Here's how the part is built. I have some questions about the finished solid (model axes, mm). Face numbers are marked on the shaded views. A direction names the side the tool comes from. Give positions to 0.01 mm unless a question says otherwise; leave off trailing zeros. Loops run counter-clockwise (first coordinate to the right, second up) from the corner with the lowest first, then second, coordinate; pieces in that order, holes last. Notation, with made-up numbers: (68.25, 23) - (88.25, 23) arc R25 ccw to (88.25, 36) - close; hole circle Ø6 at (26.5, 48). An arc over 180 degrees is marked (long way). Use a Markdown table: item, result.
from build123d import *

# Parameters (mm, degrees)
F1_R     = 28.05
F1_R_2   = 6.55
F2_DEPTH = 5
F3_SIZE  = 1
F5_DEPTH = 5.001


with BuildPart() as f2:
    # F1 (on Top) → F2 (new body)
    with BuildSketch(Plane.XY):
        Circle(F1_R)
        Circle(F1_R_2, mode=Mode.SUBTRACT)
    extrude(amount=F2_DEPTH)

    # F3
    f3_edges = [f2.edges().sort_by_distance(p)[0] for p in [
        (-28.05, 0, 0),
        (-28.05, 0, 5),
        (-6.55, 0, 5),
        (-6.55, 0, 0),
    ]]
    chamfer(f3_edges, length=F3_SIZE)

    # F4 (on face) → F5 (cut, through all)
    with BuildSketch(Plane.XY.offset(5)):
        with BuildLine():
            Line((4.0373102115, 9.746929068), (9.2035365484, 22.2193027569))
            ThreePointArc((9.2035365484, 22.2193027569), (0, 24.05), (-9.2035365484, 22.2193027569))
            Line((-9.2035365484, 22.2193027569), (-4.0373102115, 9.746929068))
            ThreePointArc((-4.0373102115, 9.746929068), (0, 10.55), (4.0373102115, 9.746929068))
        make_face()
        with BuildLine():
            ThreePointArc((-14.6407123677, 19.080147834), (-20.827910961, 12.025), (-23.844248916, 3.1391549229))
            Line((-23.844248916, 3.1391549229), (-10.4597432875, 1.3770513279))
            ThreePointArc((-10.4597432875, 1.3770513279), (-9.1365680099, 5.275), (-6.422433076, 8.3698777401))
            Line((-6.422433076, 8.3698777401), (-14.6407123677, 19.080147834))
        make_face()
        with BuildLine():
            ThreePointArc((-23.844248916, -3.1391549229), (-20.827910961, -12.025), (-14.6407123677, -19.080147834))
            Line((-14.6407123677, -19.080147834), (-6.422433076, -8.3698777401))
            ThreePointArc((-6.422433076, -8.3698777401), (-9.1365680099, -5.275), (-10.4597432875, -1.3770513279))
            Line((-10.4597432875, -1.3770513279), (-23.844248916, -3.1391549229))
        make_face()
        with BuildLine():
            ThreePointArc((-9.2035365484, -22.2193027569), (0, -24.05), (9.2035365484, -22.2193027569))
            Line((9.2035365484, -22.2193027569), (4.0373102115, -9.746929068))
            ThreePointArc((4.0373102115, -9.746929068), (0, -10.55), (-4.0373102115, -9.746929068))
            Line((-4.0373102115, -9.746929068), (-9.2035365484, -22.2193027569))
        make_face()
        with BuildLine():
            ThreePointArc((14.6407123677, -19.080147834), (20.827910961, -12.025), (23.844248916, -3.1391549229))
            Line((23.844248916, -3.1391549229), (10.4597432875, -1.3770513279))
            ThreePointArc((10.4597432875, -1.3770513279), (9.1365680099, -5.275), (6.422433076, -8.3698777401))
            Line((6.422433076, -8.3698777401), (14.6407123677, -19.080147834))
        make_face()
        with BuildLine():
            ThreePointArc((23.844248916, 3.1391549229), (20.827910961, 12.025), (14.6407123677, 19.080147834))
            Line((14.6407123677, 19.080147834), (6.422433076, 8.3698777401))
            ThreePointArc((6.422433076, 8.3698777401), (9.1365680099, 5.275), (10.4597432875, 1.3770513279))
            Line((10.4597432875, 1.3770513279), (23.844248916, 3.1391549229))
        make_face()
    extrude(amount=-F5_DEPTH, mode=Mode.SUBTRACT)


solid = f2.part
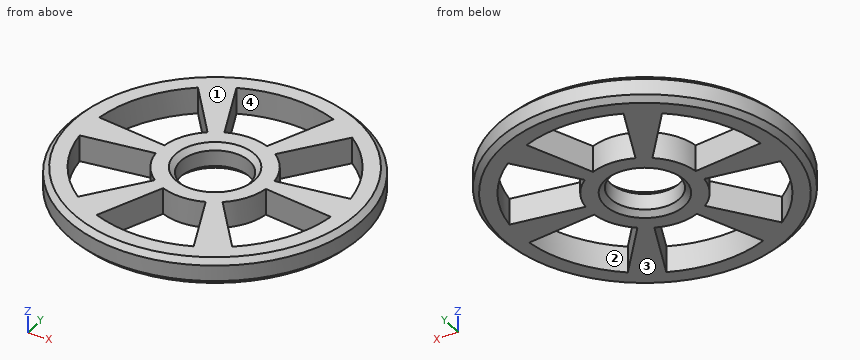
(1) Suppose I cut it at C-C on y = 0. Write out the boundary of the cut face in (x, z).
A:
| item | result |
|---|---|
| outline | (-28.05, 1) - (-27.05, 0) - (-7.55, 0) - (-6.55, 1) - (-6.55, 4) - (-7.55, 5) - (-27.05, 5) - (-28.05, 4) - close; (6.55, 1) - (7.55, 0) - (27.05, 0) - (28.05, 1) - (28.05, 4) - (27.05, 5) - (7.55, 5) - (6.55, 4) - close |
(2) If I drill on line 1 (Y direction, x = 0, z = 2.35); line 2 (Y direction, x = 15, z = 2.5); line 3 (Y direction, x = -11.5, z = 1.45), over which ranges is the centre line in solid material (lowest first)?
A:
| item | result |
|---|---|
| line 1 | -28.05 to -24.05, -10.55 to -6.55, 6.55 to 10.55, 24.05 to 28.05 |
| line 2 | -23.7 to -18.8, -1.97 to 1.97, 18.8 to 23.7 |
| line 3 | -25.58 to -14.99, -1.51 to 1.51, 14.99 to 25.58 |
(3) Suppose I cut it at A-A on z = 1.7. Write out the boundary of the cut face in (x, y), plus the area to 3 significant figures.
A:
| item | result |
|---|---|
| outline | circle Ø56.1 at (0, 0); hole (-23.84, -3.14) arc R24.05 ccw to (-14.64, -19.08) - (-6.42, -8.37) arc R10.55 cw to (-10.46, -1.38) - close; hole (-23.84, 3.14) - (-10.46, 1.38) arc R10.55 cw to (-6.42, 8.37) - (-14.64, 19.08) arc R24.05 ccw to start; hole (-9.2, -22.22) arc R24.05 ccw to (9.2, -22.22) - (4.04, -9.75) arc R10.55 cw to (-4.04, -9.75) - close; hole (-9.2, 22.22) - (-4.04, 9.75) arc R10.55 cw to (4.04, 9.75) - (9.2, 22.22) arc R24.05 ccw to start; hole circle Ø13.1 at (0, 0); hole (6.42, -8.37) - (14.64, -19.08) arc R24.05 ccw to (23.84, -3.14) - (10.46, -1.38) arc R10.55 cw to start; hole (6.42, 8.37) arc R10.55 cw to (10.46, 1.38) - (23.84, 3.14) arc R24.05 ccw to (14.64, 19.08) - close |
| area | 1,240 mm2 |
(4) Suppose I cut it at B-B on x = 0. Write out the boundary of the cut face in (y, z).
A:
| item | result |
|---|---|
| outline | (-28.05, 1) - (-27.05, 0) - (-24.05, 0) - (-24.05, 5) - (-27.05, 5) - (-28.05, 4) - close; (-10.55, 0) - (-7.55, 0) - (-6.55, 1) - (-6.55, 4) - (-7.55, 5) - (-10.55, 5) - close; (6.55, 1) - (7.55, 0) - (10.55, 0) - (10.55, 5) - (7.55, 5) - (6.55, 4) - close; (24.05, 0) - (27.05, 0) - (28.05, 1) - (28.05, 4) - (27.05, 5) - (24.05, 5) - close |
(5) On a 3-axis mill with a long thin cutter (end or side, diameter ignored), from which of +Z, -Z, +X, -X, +Y, -Y can I reach the whole of each face in a straight line? I mean the marked faces 1 and 2. Say none if no direction works.
A:
| item | result |
|---|---|
| face 1 | +Z, +X, -X, +Y, -Y |
| face 2 | +Z, -Z |
(6) We'd pull the mould along Y, two halves only. Please class the marked faces 3 and 4: pulls with the +Y half, pulls with the -Y half, needs draft (parallel to the pull), parting line crosses it, or undercut.
A:
| item | result |
|---|---|
| face 3 | needs draft |
| face 4 | undercut |
(7) Suppose I cut it at D-D on y = 15. Count the separate pieces of the cut face and the enclosed holes in it, plus the area to 3 significant figures.
A:
| item | result |
|---|---|
| separate pieces | 4 |
| enclosed holes | 0 |
| area | 99.6 mm2 |
(8) Will these pins go through, and if not, where does the flat tip stop? pin 1 (1.5 mm diameter, centred on x = -2.5, z = 4, fed in from +Y); pin 2 (1.5 mm diameter, centred on y = 19, z = 2.5, fed in from +X).
A:
| item | result |
|---|---|
| pin 1 | y = 28 |
| pin 2 | x = 21.3 |
